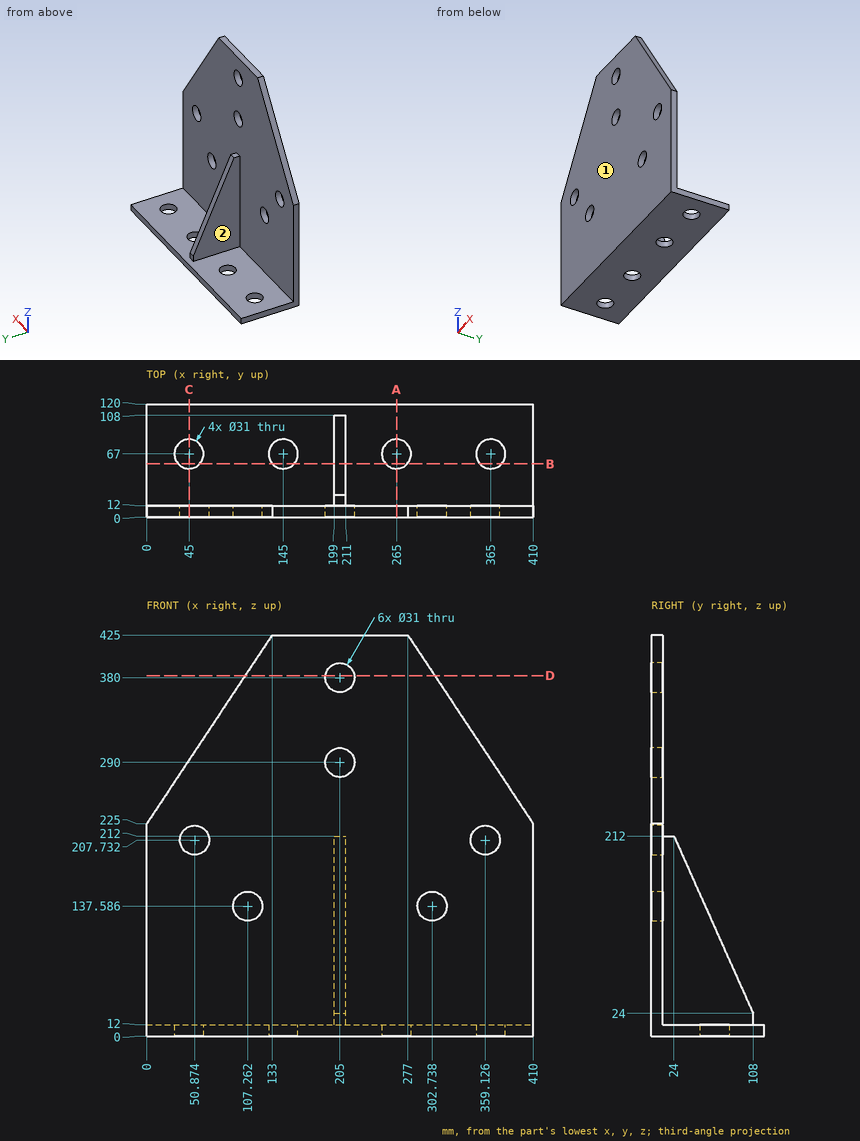
Print and shaded views of the part. All mm, measured from the part's lowest x, y and z. A direction names the side the tool comes from. Give positions to 0.01 mm unless a question says otherwise; leave off trailing zeros. Order: outer loops, then holes, each group sorted by start corner. A loop starts at its lowest first (then second) coordinate and runs counter-clockwise, first axis right, second up. Notation, with made-up numbers: (4.5, 36.25) - (16.5, 36.25) arc R25 ccw to (16.5, 74.25) - close; hole circle Ø11 at (-11.5, 88). An arc over 180 degrees is marked (long way). Use a Markdown table: item, result.
1) Saw through at D-D on z = 382. List the corners of the cut face in (x, y) (1 decimal).
Checked values:
| item | result |
|---|---|
| outline | (104.4, 0) - (189.6, 0) - (189.6, 12) - (104.4, 12) - close; (220.4, 0) - (305.6, 0) - (305.6, 12) - (220.4, 12) - close |
2) 3-axis set-ups, long thin cutter, end or side, ignore diameter. For the marked faces 1 and 2: which of +Z, -Z, +X, -X, +Y, -Y reach the whole face in a straight line?
Checked values:
| item | result |
|---|---|
| face 1 | +Z, -Z, +X, -X, -Y |
| face 2 | +Z, -X, +Y |
3) Flat gauge pins, fed straight in: P1, Ø9.5, axis at x = 203.5, z = 19, coming from the +Y side; P2, Ø3, axis at y = 60, z = 106.5, coming from the +X side. Where does each tip first touch, or does it go through?
Checked values:
| item | result |
|---|---|
| P1 | y = 108 |
| P2 | x = 211 |
4) Saw through at B-B on y = 56.5. List the corners of the cut face in (x, z), plus the area to 3 significant figures.
Checked values:
| item | result |
|---|---|
| outline | (0, 0) - (33.6, 0) - (33.6, 12) - (0, 12) - close; (56.4, 0) - (133.6, 0) - (133.6, 12) - (56.4, 12) - close; (156.4, 0) - (253.6, 0) - (253.6, 12) - (211, 12) - (211, 139.26) - (199, 139.26) - (199, 12) - (156.4, 12) - close; (276.4, 0) - (353.6, 0) - (353.6, 12) - (276.4, 12) - close; (376.4, 0) - (410, 0) - (410, 12) - (376.4, 12) - close |
| area | 5,350 mm² |
5) Probe L1, parallel to Y at x = 265, z = 5; L2, parallel to Y at x = 110, z = 201.5. List the from-to ranges inside material, lowest first. Write a range as from..to.
Checked values:
| item | result |
|---|---|
| L1 | 0..51.5, 82.5..120 |
| L2 | 0..12 |
6) Saw through at C-C on x = 45. List the corners of the cut face in (y, z).
Checked values:
| item | result |
|---|---|
| outline | (0, 0) - (51.5, 0) - (51.5, 12) - (12, 12) - (12, 193.39) - (0, 193.39) - close; (0, 222.08) - (12, 222.08) - (12, 292.67) - (0, 292.67) - close; (82.5, 0) - (120, 0) - (120, 12) - (82.5, 12) - close |
7) Saw through at A-A on x = 265. List the corners of the cut face in (y, z), plus the area to 3 significant figures.
Checked values:
| item | result |
|---|---|
| outline | (0, 0) - (51.5, 0) - (51.5, 12) - (12, 12) - (12, 425) - (0, 425) - close; (82.5, 0) - (120, 0) - (120, 12) - (82.5, 12) - close |
| area | 6,020 mm² |
